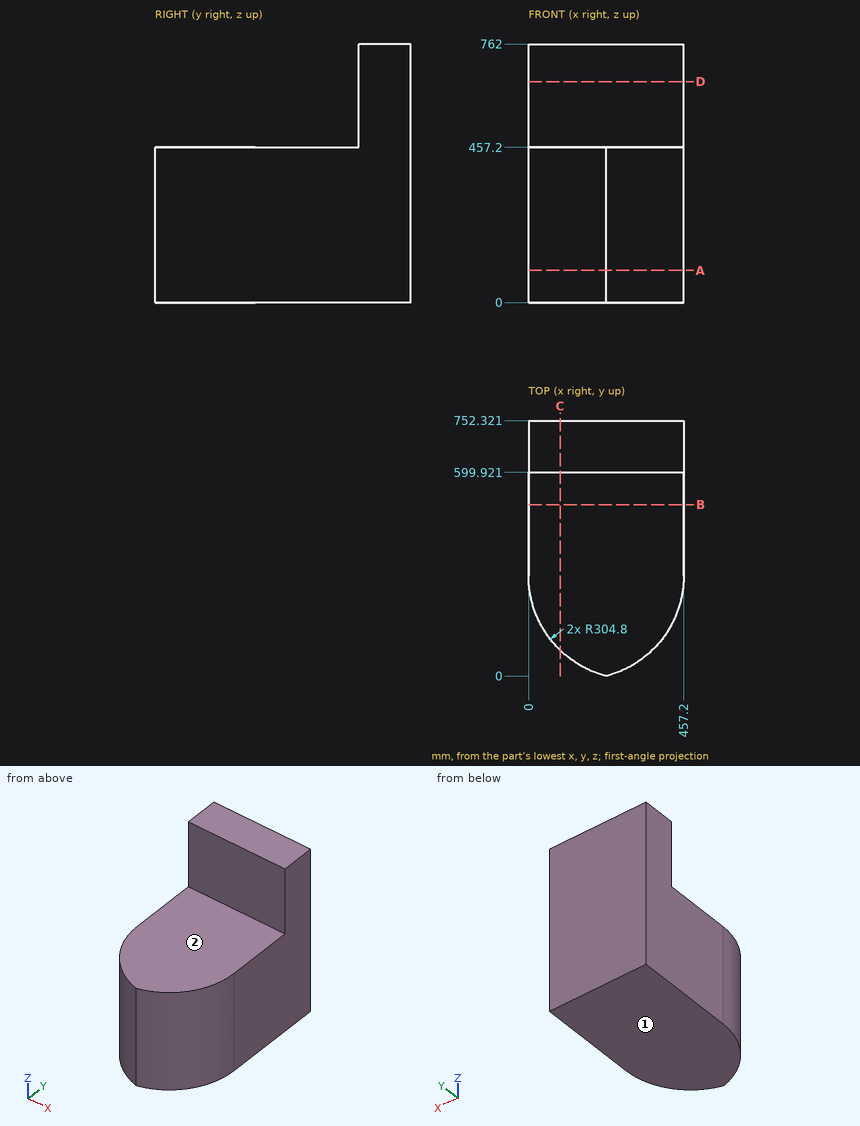
Job drawing, mm, ordinate dimensions from the low corner. One solid piece. A direction names the side the tool comes from. Give positions to 0.01 mm unless a question says otherwise; leave off trailing zeros. Write each loop counter-clockwise with the first axis right and the second up, starting at its lowest first coordinate (ties: lowest second). Pieces come first, ordered by that corner, then holes. Notation, with made-up numbers: M -19.5,11.25 L 8.5,11.25 A12 cw 8.5,29.25 Z; hole C 44.25,-4.5 d3. An arc over 180 degrees is marked long. One line per item, written item: value. Start each with the question number.
Q1. Saw through at D-D, the plane z = 651.5. Write the cut outline in (x, y).
Q2. Drop a flat-ended pin along its axis: pin 1 Ø5 at (x, z) = (364, 103) entering from -Y (1 decimal). Give the stop position or say it passes through.
Q3. Saw through at B-B, the plane y = 505. Write the cut outline in (x, z).
Q4. Saw through at A-A, the plane z = 95. Write the cut outline in (x, y), plus the area to 3 significant figures.
Q5. Probe probe 1 along Z at (x, y) = (79.5, 145.5); probe 2 along Y at (x, z) = (275, 500); probe 3 along Y at (x, z) = (191.5, 239.5). List the from-to ranges inside material, lowest first. Write a range as [from, to].
Q6. 3-axis set-ups, long thin cutter, end or side, ignore diameter. For the marked faces 1 and 2: which of +Z, -Z, +X, -X, +Y, -Y reach the whole face in a straight line?
Q7. Saw through at C-C, the plane x = 93. Write the cut outline in (y, z).
Output values:
1. outline: M 0,599.92 L 457.2,599.92 L 457.2,752.32 L 0,752.32 Z
2. pin 1: stops at y = 73.4
3. outline: M 0,0 L 457.2,0 L 457.2,457.2 L 0,457.2 Z
4. outline: M 0,295.12 A304.8 ccw 228.6,0 A304.8 ccw 457.2,295.12 L 457.2,752.32 L 0,752.32 Z
4. area: 309,000 mm²
5. probe 1: z = [0, 457.2]
5. probe 2: y = [599.92, 752.32]
5. probe 3: y = [12.16, 752.32]
6. face 1: -Z, +X, -X, +Y, -Y
6. face 2: +Z, +X, -X, -Y
7. outline: M 75.93,0 L 752.32,0 L 752.32,762 L 599.92,762 L 599.92,457.2 L 75.93,457.2 Z
